Input: part model. Units: mm. Frame: model coordinates. Round coordinates to 2 decimals unless told otherwise and drop trailing zeros. Answer as CSV lines item,"result". Start each with the question number.
1) Line query: L1, parallel to Y at x = 42, z = 0.15; L2, parallel to X at y = 42.5, z = 0.85; L3, parallel to X at y = 86, z = 0.9. Output: solid intervals per line, ascending.
2) Section query A-A, the plane z = 0.7. State how many separate pieces and enclosed holes the cut face has, and give its area (3 significant figures).
3) Mould query, pull axis X, two halves, no side actions, for faces 1 (the face through (84.353, 87.638, 0.784)), 2 (the face through (69, 89, 0)), 3 (the face through (8.96, 8.72, 0.78)), 4 (the face through (166.04, 166.28, 0.78)). Classes: +X half, -X half, draft (parallel to the pull), parting line (faces both ways), or undercut.
```python
from build123d import *

# Parameters (mm, degrees)
MODEL_R             = 3.15
BOSS_EXTRUDE1_DEPTH = 1.59


with BuildPart() as part:
    # Model → Boss-Extrude1 (new body)
    with BuildSketch(Plane.XY):
        Polygon((0, 17.67766953), (0, 157.32233047), (17.67766953, 175), (157.32233047, 175), (175, 157.32233047), (175, 17.67766953), (157.32233047, 0), (17.67766953, 0), align=None)
        with Locations((87.5, 87.5)):
            Circle(MODEL_R, mode=Mode.SUBTRACT)
        Polygon((139.381727984, 47.639087297), (140.795941546, 46.224873734), (140.088834765, 45.517766953), (138.674621202, 46.931980515), align=None, mode=Mode.SUBTRACT)
        Polygon((135.139087297, 43.396446609), (136.553300859, 41.982233047), (135.846194078, 41.275126266), (134.431980515, 42.689339828), align=None, mode=Mode.SUBTRACT)
        Polygon((132.310660172, 40.568019485), (133.724873734, 39.153805922), (133.017766953, 38.446699141), (131.603553391, 39.860912703), align=None, mode=Mode.SUBTRACT)
        Polygon((128.068019485, 36.325378798), (129.482233047, 34.911165235), (128.775126266, 34.204058454), (127.360912703, 35.618272016), align=None, mode=Mode.SUBTRACT)
        Polygon((87.853553391, 76.539844892), (89.267766953, 75.125631329), (88.560660172, 74.418524548), (87.146446609, 75.83273811), align=None, mode=Mode.SUBTRACT)
        Polygon((92.096194078, 80.782485579), (93.51040764, 79.368272016), (92.803300859, 78.661165235), (91.389087297, 80.075378798), align=None, mode=Mode.SUBTRACT)
        Polygon((47.639087297, 35.618272016), (46.224873734, 34.204058454), (45.517766953, 34.911165235), (46.931980515, 36.325378798), align=None, mode=Mode.SUBTRACT)
        Polygon((43.396446609, 39.860912703), (41.982233047, 38.446699141), (41.275126266, 39.153805922), (42.689339828, 40.568019485), align=None, mode=Mode.SUBTRACT)
        Polygon((40.568019485, 42.689339828), (39.153805922, 41.275126266), (38.446699141, 41.982233047), (39.860912703, 43.396446609), align=None, mode=Mode.SUBTRACT)
        Polygon((36.325378798, 46.931980515), (34.911165235, 45.517766953), (34.204058454, 46.224873734), (35.618272016, 47.639087297), align=None, mode=Mode.SUBTRACT)
        Polygon((75.83273811, 86.439339828), (74.418524548, 85.025126266), (73.711417767, 85.732233047), (75.125631329, 87.146446609), align=None, mode=Mode.SUBTRACT)
        Polygon((80.075378798, 82.196699141), (78.661165235, 80.782485579), (77.954058454, 81.48959236), (79.368272016, 82.903805922), align=None, mode=Mode.SUBTRACT)
        Polygon((82.903805922, 79.368272016), (81.48959236, 77.954058454), (80.782485579, 78.661165235), (82.196699141, 80.075378798), align=None, mode=Mode.SUBTRACT)
        Polygon((87.146446609, 75.125631329), (85.732233047, 73.711417767), (85.025126266, 74.418524548), (86.439339828, 75.83273811), align=None, mode=Mode.SUBTRACT)
        Polygon((101.288582233, 89.267766953), (99.874368671, 87.853553391), (99.16726189, 88.560660172), (100.581475452, 89.974873734), align=None, mode=Mode.SUBTRACT)
        Polygon((97.045941546, 93.51040764), (95.631727984, 92.096194078), (94.924621202, 92.803300859), (96.338834765, 94.217514421), align=None, mode=Mode.SUBTRACT)
        Polygon((94.217514421, 96.338834765), (92.803300859, 94.924621202), (92.096194078, 95.631727984), (93.51040764, 97.045941546), align=None, mode=Mode.SUBTRACT)
        Polygon((89.974873734, 100.581475452), (88.560660172, 99.16726189), (87.853553391, 99.874368671), (89.267766953, 101.288582233), align=None, mode=Mode.SUBTRACT)
        Polygon((129.482233047, 140.088834765), (128.068019485, 138.674621202), (127.360912703, 139.381727984), (128.775126266, 140.795941546), align=None, mode=Mode.SUBTRACT)
        Polygon((133.724873734, 135.846194078), (132.310660172, 134.431980515), (131.603553391, 135.139087297), (133.017766953, 136.553300859), align=None, mode=Mode.SUBTRACT)
        Polygon((136.553300859, 133.017766953), (135.139087297, 131.603553391), (134.431980515, 132.310660172), (135.846194078, 133.724873734), align=None, mode=Mode.SUBTRACT)
        Polygon((140.795941546, 128.775126266), (139.381727984, 127.360912703), (138.674621202, 128.068019485), (140.088834765, 129.482233047), align=None, mode=Mode.SUBTRACT)
        Polygon((94.924621202, 83.610912703), (96.338834765, 82.196699141), (95.631727984, 81.48959236), (94.217514421, 82.903805922), align=None, mode=Mode.SUBTRACT)
        Polygon((99.16726189, 87.853553391), (100.581475452, 86.439339828), (99.874368671, 85.732233047), (98.460155108, 87.146446609), align=None, mode=Mode.SUBTRACT)
        Polygon((75.125631329, 89.267766953), (76.539844892, 87.853553391), (75.83273811, 87.146446609), (74.418524548, 88.560660172), align=None, mode=Mode.SUBTRACT)
        Polygon((79.368272016, 93.51040764), (80.782485579, 92.096194078), (80.075378798, 91.389087297), (78.661165235, 92.803300859), align=None, mode=Mode.SUBTRACT)
        Polygon((82.196699141, 96.338834765), (83.610912703, 94.924621202), (82.903805922, 94.217514421), (81.48959236, 95.631727984), align=None, mode=Mode.SUBTRACT)
        Polygon((86.439339828, 100.581475452), (87.853553391, 99.16726189), (87.146446609, 98.460155108), (85.732233047, 99.874368671), align=None, mode=Mode.SUBTRACT)
        Polygon((34.204058454, 130.189339828), (35.618272016, 128.775126266), (34.911165235, 128.068019485), (33.496951673, 129.482233047), align=None, mode=Mode.SUBTRACT)
        Polygon((38.446699141, 134.431980515), (39.860912703, 133.017766953), (39.153805922, 132.310660172), (37.73959236, 133.724873734), align=None, mode=Mode.SUBTRACT)
        Polygon((41.275126266, 137.26040764), (42.689339828, 135.846194078), (41.982233047, 135.139087297), (40.568019485, 136.553300859), align=None, mode=Mode.SUBTRACT)
        Polygon((45.517766953, 141.503048327), (46.931980515, 140.088834765), (46.224873734, 139.381727984), (44.810660172, 140.795941546), align=None, mode=Mode.SUBTRACT)
    extrude(amount=BOSS_EXTRUDE1_DEPTH)


solid = part.part
```
Findings:
1,L1,"y = 0 to 38.46, 39.88 to 135.16, 136.54 to 175"
1,L2,"x = 0 to 38.96, 40.38 to 134.62, 136.04 to 175"
1,L3,"x = 0 to 73.98, 75.39 to 84.73, 90.27 to 99.61, 100.14 to 175"
2,separate pieces,"1"
2,enclosed holes,"33"
2,area,"29,900 mm^2"
3,face 1,"undercut"
3,face 2,"draft"
3,face 3,"-X half"
3,face 4,"+X half"
